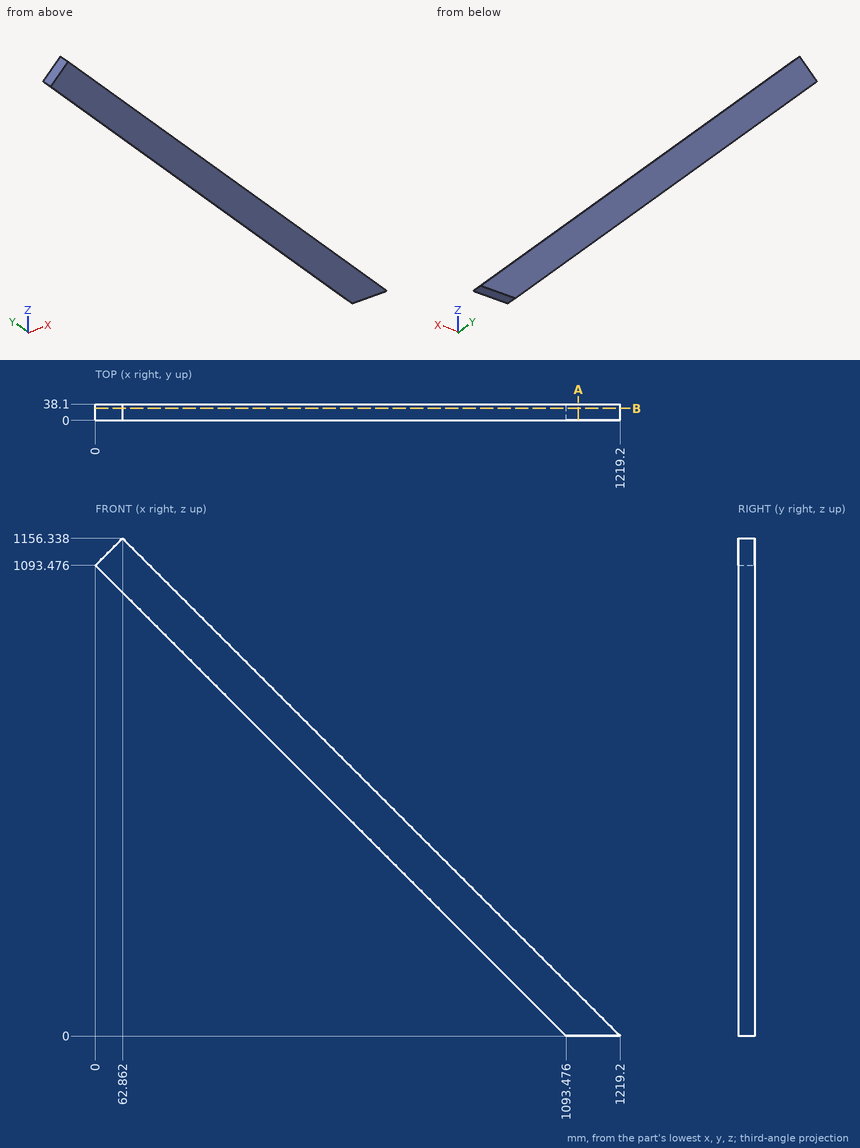
Answer from the drawing. Dimensions are ordinates in mm from the lowest x, y and z of the part. Coordinates: 2 decimals unless noted, no trailing zeros. Write each loop counter-clockwise with the first axis right and the second up, starting at its lowest first coordinate (ties: lowest second). Pieces come first, ordered by that corner, then holes. Notation, with made-up numbers: M 72,-34 L 78,-34 A12 ccw 78,-17 Z; hole C -6,19.25 d6. An arc over 180 degrees is marked long. Put each result on its own line as item: value. Start each with the question number.
1. Flat-ended cylindrical pins translate along their axes: P1, Ø3, axis at x = 694, y = 32.5, coming from the -Z side (1 decimal); P2, Ø1.5, axis at y = 8.5, z = 199, coming from the -X side (1 decimal); P3, Ø1.5, axis at x = 473.5, y = 27.5, coming from the -Z side (1 decimal). Find the tip coordinate at first contact, or state that the pin passes through.
2. A cutting plane is placed at A-A on x = 1122. Write down the section's boundary in (y, z).
3. A cutting plane is placed at B-B on y = 28. Write down the section's boundary in (x, z), then the cut area to 3 significant figures.
4. Consider line 1 (X direction, y = 5, z = 150.5) (1 decimal); line 2 (X direction, y = 2.5, z = 882.5) (1 decimal); line 3 (Z direction, x = 69, y = 35) (1 decimal). Determine where each line is inside the solid, lowest interval first. Write a range as from..to.
Resolved:
1. P1: stops at z = 398
1. P2: stops at x = 893.7
1. P3: stops at z = 619.2
2. outline: M 0,0 L 38.1,0 L 38.1,97.2 L 0,97.2 Z
3. outline: M 0,1093.48 L 1093.48,0 L 1219.2,0 L 62.86,1156.34 Z
3. area: 141,000 mm2
4. line 1: x = 943..1068.7
4. line 2: x = 211..336.7
4. line 3: z = 1024.5..1150.2
